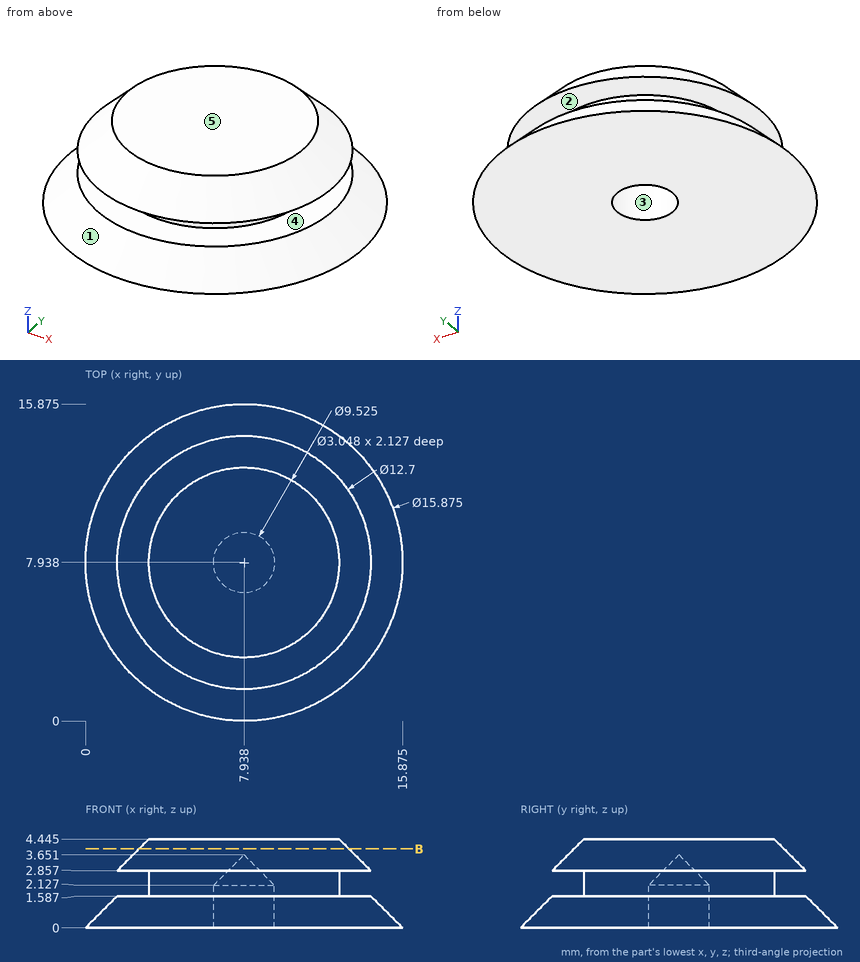
Check sheet for the drawn part. Datum: minimum x, y, z corner. Units: mm. A direction names the side the tool comes from. Round coordinates to 2 decimals unless told otherwise and drop trailing zeros. Write each loop counter-clockwise with the first axis right and the second up, starting at its lowest first coordinate (ties: lowest second). Pieces come first, ordered by that corner, then holes. Notation, with made-up numbers: (55, 31) -> (68, 31) arc R22 ccw to (68, 68) -> close; hole circle Ø3 at (-29, 12). An arc over 180 degrees is marked (long way). One line per item, written item: value. Start each with the question number.
(1) Access from +Z, -Z, +X, -X, +Y, -Y to the whole of each face (thin tool, end or side, straight path). Record for the marked faces 1 and 2.
(2) Scan lines: line 1 (Z direction, x = 7.75, y = 2) (1 decimal); line 2 (Y direction, x = 7, z = 2.6) (1 decimal); line 3 (Y direction, x = 3.75, z = 3.1) (1 decimal). Record each from-to range of solid material in increasing order. Write a range as [from, to].
(3) Cross-section at B-B, the plane z = 3.95. Record the cut outline in (x, y) (1 decimal).
(4) Go/stop test with flat-tipped pins: pin 1 Ø4 at (x, y) = (12.5, 2.5) entering from +Z; pin 2 Ø2 at (x, z) = (11.5, 2.5) entering from -Y; pin 3 Ø2.5 at (x, y) = (7.94, 7.94) entering from -Z. Record where each tip stops, or that it passes through.
(5) Draft check along Z on the marked faces 3, 4 and 5. Enter one of: +Z half, -Z half, draft (parallel to the pull), parting line (faces both ways), or undercut.
Answer:
1. face 1: +Z
1. face 2: none
2. line 1: [0, 1.6], [2.9, 3.3]
2. line 2: [3.3, 7.5], [8.4, 12.6]
2. line 3: [3.5, 12.4]
3. outline: circle Ø10.5 at (7.9, 7.9)
4. pin 1: z = 4.11
4. pin 2: y = 2.16
4. pin 3: z = 2.4
5. face 3: draft
5. face 4: undercut
5. face 5: +Z half
